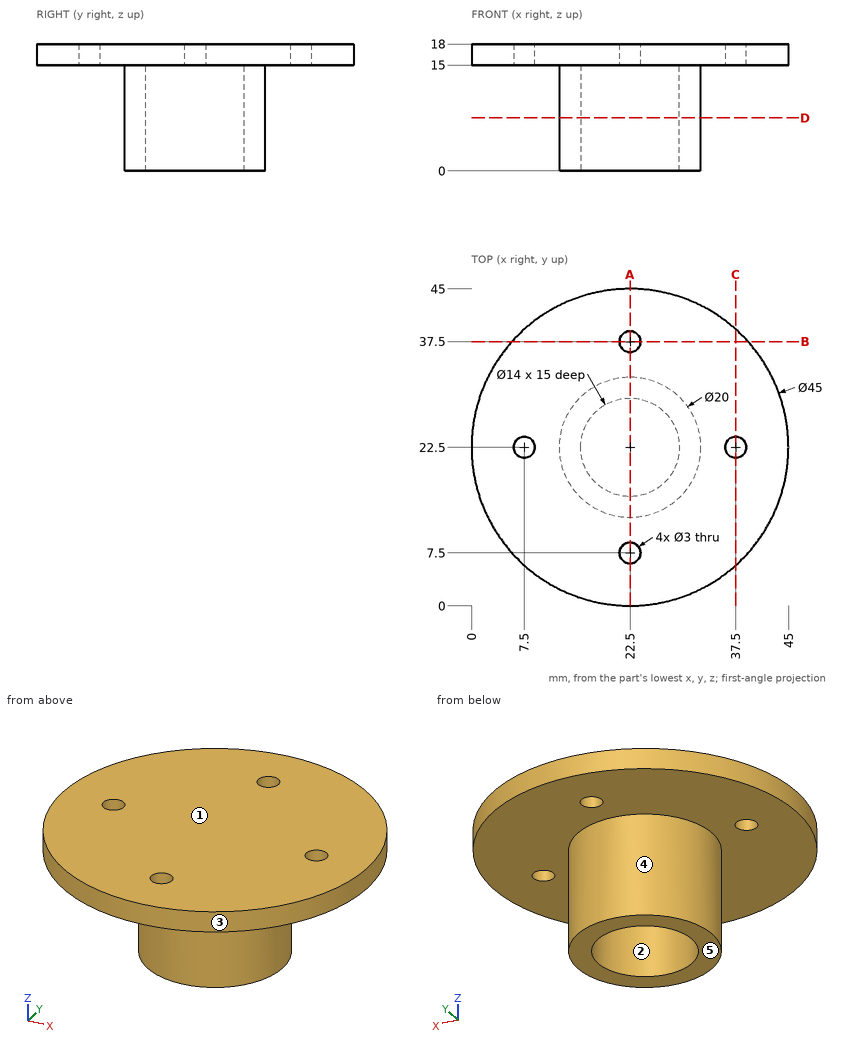
Could you check a few things on this drawing? It's one solid part, dimensions in mm from its lowest x, y, z. A direction names the side the tool comes from. Coordinates: 2 decimals unless noted, no trailing zeros. Loops run counter-clockwise (first coordinate to the right, second up) from the corner with the lowest first, then second, coordinate; pieces in that order, holes last. Notation, with made-up numbers: (74, 51) - (106, 51) arc R19 ccw to (106, 59) - close; hole circle Ø10 at (-38, 37.5). An arc over 180 degrees is marked (long way). Return JSON: item names as keys, results as strings. Group by question number.
Item 1: We'd pull the mould along X, two halves only. Please class the marked faces 1, 2 and 3: +X half, -X half, draft (parallel to the pull), parting line (faces both ways), or undercut.
Item 2: On a 3-axis mill with a long thin cutter (end or side, diameter ignored), from which of +Z, -Z, +X, -X, +Y, -Y can I reach the whole of each face in a straight line? I mean the marked faces 4 and 5. Say none if no direction works.
Item 3: If we section it at A-A on x = 22.5: Write out the boundary of the cut face in (y, z).
Item 4: Will these pins go through, and if not, where does the flat tip stop? P1, Ø1.8, axis at x = 22.5, y = 37.5, coming from the +Z side; P2, Ø5, axis at x = 37.5, y = 22.5, coming from the -Z side; P3, Ø3, axis at x = 24.5, z = 4, coming from the +Y side; P4, Ø3, axis at x = 20.5, z = 13, coming from the -Y side.
Item 5: I need wall thicknesses on line 1 (Y direction, x = 22.5, z = 16); line 2 (Y direction, x = 22.5, z = 7.75); line 3 (Z direction, x = 10, y = 11). Which ranges of each line are inside material? Lowest first, please. Write a range as from..to.
Item 6: If we section it at D-D on z = 7.5: Write out the boundary of the cut face in (x, y).
Item 7: If we section it at B-B on y = 37.5: Write out the boundary of the cut face in (x, z), and give its area (3 significant figures).
Calculated:
{
 "1": {"face 1": "draft", "face 2": "undercut", "face 3": "parting line"},
 "2": {"face 4": "-Z", "face 5": "-Z, +X, -X, +Y, -Y"},
 "3": {"outline": "(0, 15) - (6, 15) - (6, 18) - (0, 18) - close; (9, 15) - (12.5, 15) - (12.5, 0) - (15.5, 0) - (15.5, 15) - (29.5, 15) - (29.5, 0) - (32.5, 0) - (32.5, 15) - (36, 15) - (36, 18) - (9, 18) - close; (39, 15) - (45, 15) - (45, 18) - (39, 18) - close"},
 "4": {"P1": "passes through", "P2": "stops at z = 15", "P3": "stops at y = 32.49", "P4": "stops at y = 12.51"},
 "5": {"line 1": "y = 0..6, 9..36, 39..45", "line 2": "y = 12.5..15.5, 29.5..32.5", "line 3": "z = 15..18"},
 "6": {"outline": "circle Ø20 at (22.5, 22.5); hole circle Ø14 at (22.5, 22.5)"},
 "7": {"outline": "(5.73, 15) - (21, 15) - (21, 18) - (5.73, 18) - close; (24, 15) - (39.27, 15) - (39.27, 18) - (24, 18) - close", "area": "91.6 mm^2"}
}
